Can you work these out from the model? Positions are in its coordinate system, mm. Round coordinates to 2 decimals unless told otherwise and drop trailing zeros. Write each loop counter-clockwise with the first axis right and the second up, starting at its lowest first coordinate (ties: lowest second). Pieces come first, ordered by that corner, then holes. Notation, with made-up numbers: (14, 81.25) - (53, 81.25) arc R21 cw to (53, 89.25) - close; hole circle Ø1 at (56, -13). An arc over 180 degrees is marked (long way). One line per item, written item: value. Start each with the question number.
(1) If I drill on L1, parallel to Y at x = 200.5, z = 0.35; L2, parallel to X at y = 7, z = 0.45; L3, parallel to X at y = 8, z = 0.7, over which ranges is the centre line in solid material (lowest first)? Write a range as from..to.
(2) I want a section at B-B on y = 48. List the corners of the cut face in (x, z) for me, plus the area to 3 significant figures.
(3) I'm going to push a flat-ended pin straight in: pin 1 Ø4 at (x, y) = (-116.05, -2.06) entering from +Z. Where does the tip first touch, or does it pass through?
(4) I want a section at A-A on z = 0.65. Give the number of separate pieces and of enclosed holes in the cut face, plus the area to 3 significant figures.
from build123d import *

# Parameters (mm, degrees)
F1_DEPTH       = 0.9144
F3_D           = 3.556
F3_CSINK_D     = 4.826
F3_CSINK_ANGLE = 100


with BuildPart() as f1:
    # F0 (on Top) → F1 (new body)
    with BuildSketch(Plane.XY):
        with BuildLine():
            ThreePointArc((-241.3, 63.5), (-304.8, 0), (-241.3, -63.5))
            Line((-241.3, -63.5), (241.3, -63.5))
            ThreePointArc((241.3, -63.5), (304.8, 0), (241.3, 63.5))
            Line((241.3, 63.5), (-241.3, 63.5))
        make_face()
    extrude(amount=F1_DEPTH)

    # F3 (through all)
    with Locations(Plane.XY.offset(0.9144)):
        with Locations((-226.15525, -2.056472), (-203.80325, -2.056472), (-182.08625, -2.056472), (-159.91205, -2.056472), (-137.66165, -2.056472), (-116.04625, -2.056472), (-93.99905, -2.056472), (-71.92645, -2.056472), (-50.18405, -2.056472), (-24.96185, -2.056472), (0.1778, -2.056472), (25.4508, -2.056472), (50.546, -2.056472), (75.565, -2.056472), (100.8634, -2.056472), (125.5268, -2.056472), (150.8252, -2.056472), (175.8696, -2.056472), (200.9394, -2.056472), (226.1362, -2.056472)):
            CounterSinkHole(F3_D / 2, F3_CSINK_D / 2, counter_sink_angle=F3_CSINK_ANGLE)


solid = f1.part
Established:
1. L1: -63.5..-3.78, -0.33..63.5
1. L2: -304.41..304.41
1. L3: -304.29..304.29
2. outline: (-282.87, 0) - (282.87, 0) - (282.87, 0.91) - (-282.87, 0.91) - close
2. area: 517 mm2
3. pin 1: z = 0.57
4. separate pieces: 1
4. enclosed holes: 20
4. area: 73,700 mm2
